Design review of the part built by this model. Coordinates are the model's own, in mm. Face numbers are marked on the shaded views. A direction names the side the tool comes from. Give positions to 0.01 mm unless a question says otherwise; leave off trailing zeros. Loops run counter-clockwise (first coordinate to the right, second up) from the corner with the lowest first, then second, coordinate; pieces in that order, holes last. Notation, with made-up numbers: (87, 71) -> (107, 71) arc R26 cw to (107, 107) -> close; hole circle Ø3 at (14, 6). An arc over 180 degrees is marked (long way). Answer in a Markdown table with one row per item. Add a question column.
(1) For the marked faces 1, 2, 3, 4 and 5, list the 3-axis set-ups (+Z, -Z, +X, -X, +Y, -Y) from which the entire face can be reached by the end or side of a thin tool; tool diameter is ignored.
(2) Consider section D-D on y = 24.5. Write out the cut boundary in (x, z).
(3) Consider section C-C on z = 26.25. Write out the cut boundary in (x, y).
(4) For pin 1 (5 mm diameter, centred on x = -35, y = 14, fed in from +Z); pin 2 (8 mm diameter, centred on x = -27, y = 13, fed in from -Z); pin 3 (2 mm diameter, centred on x = -29, z = 22.5, fed in from -Y); pin 4 (1.5 mm diameter, centred on x = -48, y = 20, fed in from +Z), all flat-tipped, find the tip position at first contact; note any pin that passes through.
(5) Draft analysis for pull direction Y (two halves, no side actions). For the marked faces 6, 7 and 8, state which applies: +Y half, -Y half, draft (parallel to the pull), parting line (faces both ways), or undercut.
(6) Consider section B-B on y = 8.15. Write out the cut boundary in (x, z).
(7) For line 1 (X direction, y = 20.75, z = 11.75); line 2 (Y direction, x = -3.5, z = 14.05); line 3 (Y direction, x = -48.3, z = 14.05), list the stretches that pass through material, from the lowest coordinate up.
(8) Consider section A-A on z = 14.05. Write out the cut boundary in (x, y).
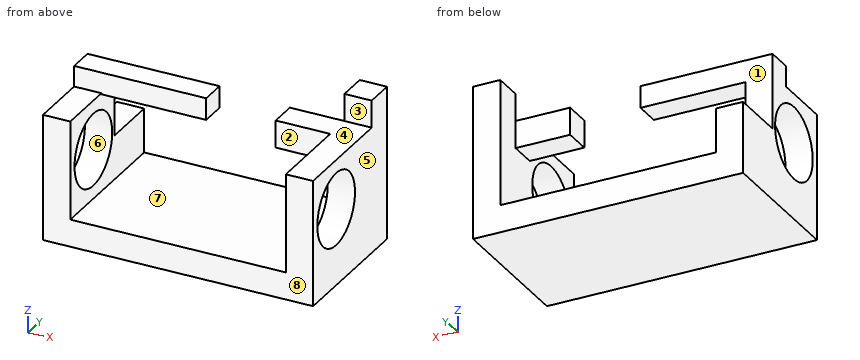
from build123d import *

# Parameters (mm, degrees)
CROQUIS2_W              = 49.5
CROQUIS2_H              = 26.9
SALIENTE_EXTRUIR1_DEPTH = 26.1
CORTAR_EXTRUIR2_DEPTH   = 26.1
CORTAR_EXTRUIR4_REACH   = 60.181
CROQUIS9_R              = 6.65
CORTAR_EXTRUIR5_REACH   = 64.089
CROQUIS8_R              = 6.65
CORTAR_EXTRUIR6_DEPTH   = 10.4
CROQUIS10_W             = 24.2
CROQUIS10_H             = 11
CORTAR_EXTRUIR7_DEPTH   = 3.8
CROQUIS13_W             = 19.2
CROQUIS13_H             = 11
CORTAR_EXTRUIR8_DEPTH   = 0.2
CORTAR_EXTRUIR9_REACH   = 64.089
CROQUIS14_W             = 3.8
CROQUIS14_H             = 20.7
CROQUIS15_W             = 10
CROQUIS15_H             = 5
SALIENTE_EXTRUIR2_DEPTH = 5
CROQUIS16_W             = 5
CROQUIS16_H             = 5.4
SALIENTE_EXTRUIR3_DEPTH = 1.2


with BuildPart() as part:
    # Croquis2 → Saliente-Extruir1 (new body)
    with BuildSketch(Plane(origin=(0, 0, 0), x_dir=(1, 0, 0), z_dir=(0, 1, 0))):
        with Locations((-24.75, -13.45)):
            Rectangle(CROQUIS2_W, CROQUIS2_H)
    extrude(amount=SALIENTE_EXTRUIR1_DEPTH)

    # Croquis6 → Cortar-Extruir2 (cut)
    with BuildSketch(Plane(origin=(0, 26.1, 0), x_dir=(1, 0, 0), z_dir=(0, 1, 0))):
        Polygon((-44.5, -21.9), (-44.5, -22.9), (-25.3, -22.9), (-25.3, -26.9), (-5, -26.9), (-5, -21.9), (-5, -5), (-44.5, -5), align=None)
    extrude(amount=-CORTAR_EXTRUIR2_DEPTH, mode=Mode.SUBTRACT)

    # Croquis9 → Cortar-Extruir4 (cut, up to next)
    with BuildSketch(Plane(origin=(-44.5, 0, 0), x_dir=(0, 0, -1), z_dir=(1, 0, 0)), mode=Mode.PRIVATE) as cortar_extruir4_sk1:
        with Locations((-14.05, 8.15)):
            Circle(CROQUIS9_R)
    cortar_extruir4_tool1 = extrude(cortar_extruir4_sk1.sketch, amount=-CORTAR_EXTRUIR4_REACH, mode=Mode.PRIVATE) & part.part
    add(cortar_extruir4_tool1.solids().sort_by_distance((-44.5, 8.15, 14.05))[0], mode=Mode.SUBTRACT)

    # Croquis8 → Cortar-Extruir5 (cut, up to next)
    with BuildSketch(Plane(origin=(0, 0, 0), x_dir=(0, 0, -1), z_dir=(1, 0, 0)), mode=Mode.PRIVATE) as cortar_extruir5_sk1:
        with Locations((-14.05, 8.15)):
            Circle(CROQUIS8_R)
    cortar_extruir5_tool1 = extrude(cortar_extruir5_sk1.sketch, amount=-CORTAR_EXTRUIR5_REACH, mode=Mode.PRIVATE) & part.part
    add(cortar_extruir5_tool1.solids().sort_by_distance((0, 8.15, 14.05))[0], mode=Mode.SUBTRACT)

    # Croquis11 → Cortar-Extruir6 (cut)
    with BuildSketch(Plane(origin=(0, 26.1, 0), x_dir=(1, 0, 0), z_dir=(0, 1, 0))):
        Polygon((-44.5, -13.1), (-49.5, -13.1), (-49.5, -26.9), (-25.3, -26.9), (-25.3, -22.9), (-44.5, -22.9), align=None)
    extrude(amount=-CORTAR_EXTRUIR6_DEPTH, mode=Mode.SUBTRACT)

    # Croquis10 → Cortar-Extruir7 (cut)
    with BuildSketch(Plane.XY.offset(26.9)):
        with Locations((-37.4, 5.5)):
            Rectangle(CROQUIS10_W, CROQUIS10_H)
    extrude(amount=-CORTAR_EXTRUIR7_DEPTH, mode=Mode.SUBTRACT)

    # Croquis13 → Cortar-Extruir8 (cut)
    with BuildSketch(Plane(origin=(0, 0, 22.9), x_dir=(-1, 0, 0), z_dir=(0, 0, -1))):
        with Locations((34.9, 5.5)):
            Rectangle(CROQUIS13_W, CROQUIS13_H)
    extrude(amount=-CORTAR_EXTRUIR8_DEPTH, mode=Mode.SUBTRACT)

    # Croquis14 → Cortar-Extruir9 (cut, up to next)
    with BuildSketch(Plane(origin=(0, 0, 0), x_dir=(0, 0, -1), z_dir=(1, 0, 0)), mode=Mode.PRIVATE) as cortar_extruir9_sk1:
        with Locations((-25, 10.35)):
            Rectangle(CROQUIS14_W, CROQUIS14_H)
    cortar_extruir9_tool1 = extrude(cortar_extruir9_sk1.sketch, amount=-CORTAR_EXTRUIR9_REACH, mode=Mode.PRIVATE) & part.part
    add(cortar_extruir9_tool1.solids().sort_by_distance((0, 10.35, 25))[0], mode=Mode.SUBTRACT)

    # Croquis15 → Saliente-Extruir2 (add)
    with BuildSketch(Plane.XY.offset(23.1)):
        with Locations((-10, 18.2)):
            Rectangle(CROQUIS15_W, CROQUIS15_H)
    extrude(amount=-SALIENTE_EXTRUIR2_DEPTH)

    # Croquis16 → Saliente-Extruir3 (add)
    with BuildSketch(Plane.XY.offset(26.9)):
        with Locations((-2.5, 23.4)):
            Rectangle(CROQUIS16_W, CROQUIS16_H)
    extrude(amount=SALIENTE_EXTRUIR3_DEPTH)


solid = part.part
Values follow:
| question | item | result |
|---|---|---|
| 1 | face 1 | +Z, -X, +Y |
| 1 | face 2 | +Z, -Y |
| 1 | face 3 | +Z, +X, -X, -Y |
| 1 | face 4 | +Z, +X, -Y |
| 1 | face 5 | +Z, -Z, +X, +Y, -Y |
| 2 | outline | (-49.5, 0) -> (0, 0) -> (0, 28.1) -> (-5, 28.1) -> (-5, 5) -> (-44.5, 5) -> (-44.5, 13.1) -> (-49.5, 13.1) -> close |
| 3 | outline | (-49.5, 11) -> (-25.3, 11) -> (-25.3, 15.7) -> (-49.5, 15.7) -> close; (-5, 20.7) -> (0, 20.7) -> (0, 26.1) -> (-5, 26.1) -> close |
| 4 | pin 1 | z = 26.9 |
| 4 | pin 2 | z = 0 |
| 4 | pin 3 | y = 11 |
| 4 | pin 4 | z = 13.1 |
| 5 | face 6 | undercut |
| 5 | face 7 | draft |
| 5 | face 8 | -Y half |
| 6 | outline | (-49.5, 0) -> (0, 0) -> (0, 7.4) -> (-5, 7.4) -> (-5, 5) -> (-44.5, 5) -> (-44.5, 7.4) -> (-49.5, 7.4) -> close; (-49.5, 20.7) -> (-44.5, 20.7) -> (-44.5, 23.1) -> (-49.5, 23.1) -> close; (-5, 20.7) -> (0, 20.7) -> (0, 23.1) -> (-5, 23.1) -> close |
| 7 | line 1 | -49.5 to -44.5, -5 to 0 |
| 7 | line 2 | 0 to 1.5, 14.8 to 26.1 |
| 7 | line 3 | 0 to 1.5, 14.8 to 15.7 |
| 8 | outline | (-49.5, 0) -> (-44.5, 0) -> (-44.5, 1.5) -> (-49.5, 1.5) -> close; (-49.5, 14.8) -> (-44.5, 14.8) -> (-44.5, 15.7) -> (-49.5, 15.7) -> close; (-5, 0) -> (0, 0) -> (0, 1.5) -> (-5, 1.5) -> close; (-5, 14.8) -> (0, 14.8) -> (0, 26.1) -> (-5, 26.1) -> close |
